The listing builds one solid part. Answer for the finished solid, in the listing's coordinates (mm). A direction names the side the tool comes from. Round coordinates to 2 decimals unless told otherwise and drop trailing zeros. Write each loop counter-clockwise with the first axis right and the second up, starting at its lowest first coordinate (ties: lowest second). Pieces come first, ordered by that corner, then holes. Notation, with made-up numbers: (63, -23) - (119, -23) arc R17 cw to (119, -1) - close; hole circle Ø2 at (-2, -23.75). An arc over 180 degrees is marked (long way). Return JSON: item names as keys, results as strings. Group by question number.
(1) Section C-C, the plane y = -91 is taken. Write down the section's boundary in (x, z), then the cut area to 3 significant figures.
(2) Each of these flat-tipped pins is pushed along its axis until it touches: pin 1 (3 mm diameter, centred on y = -12.5, z = 4.5, fed in from -X); pin 2 (3 mm diameter, centred on y = 19.5, z = 2, fed in from +X); pin 3 (6 mm diameter, centred on x = -26.5, y = -35, fed in from -Z); pin 4 (1.9 mm diameter, centred on x = -18, z = 4.5, fed in from +Y). Where does it stop, or does it pass through?
(3) Section D-D, the plane x = 32.5 is taken. Write down the section's boundary in (y, z).
(4) Section B-B, the plane x = 0 is taken. Write down the section's boundary in (y, z) (3 decimals).
(5) Find the intervals of material crossed by line 1 along X through (y, z) = (7, 3.5) (3 decimals); line 2 along X through (y, z) = (20.5, 3.25) (3 decimals); line 3 along Y through (x, z) = (110, 2), in increasing order. Write a range as [from, to].
(6) Section A-A, the plane z = 3.75 is taken. Write down the section's boundary in (x, y) (3 decimals), then the cut area to 3 significant figures.
(7) Which of the six approach directions +Z, -Z, +X, -X, +Y, -Y give full straight-line access (tool end or side, diameter ignored) to faces 1 (the flat face through (-3.175, -14, 3)), 2 (the flat face through (-2, 30, 6.35))?
(8) Determine the mould class of faces 3 (the cylindrical face through (-27.53, -123.98, 3.13)), 4 (the cylindrical face through (-28.574, -0.07, 3.131)), 5 (the flat face through (-2, 30, 0)) for opening direction Y: +Y half, -Y half, draft (parallel to the pull), parting line (faces both ways), or undercut.
```python
from build123d import *

# Parameters (mm, degrees)
F0_R     = 127
F1_DEPTH = 6.35


with BuildPart() as f1:
    # F0 (on Top) → F1 (new body)
    with BuildSketch(Plane.XY):
        Circle(F0_R)
        with BuildLine():
            Line((-3.175, -25.4), (-3.175, -3.175))
            Line((-3.175, -3.175), (-25.4, -3.175))
            ThreePointArc((-25.4, -3.175), (-28.575, 0), (-25.4, 3.175))
            Line((-25.4, 3.175), (-3.175, 3.175))
            Line((-3.175, 3.175), (-3.175, 25.4))
            ThreePointArc((-3.175, 25.4), (0, 28.575), (3.175, 25.4))
            Line((3.175, 25.4), (3.175, 3.175))
            Line((3.175, 3.175), (25.4, 3.175))
            ThreePointArc((25.4, 3.175), (28.575, 0), (25.4, -3.175))
            Line((25.4, -3.175), (3.175, -3.175))
            Line((3.175, -3.175), (3.175, -25.4))
            ThreePointArc((3.175, -25.4), (0, -28.575), (-3.175, -25.4))
        make_face(mode=Mode.SUBTRACT)
    extrude(amount=F1_DEPTH)


solid = f1.part
```
Working result:
{
 "1": {"outline": "(-88.59, 0) - (88.59, 0) - (88.59, 6.35) - (-88.59, 6.35) - close", "area": "1,130 mm^2"},
 "2": {"pin 1": "stops at x = -126.52", "pin 2": "stops at x = 125.72", "pin 3": "stops at z = 0", "pin 4": "stops at y = 125.85"},
 "3": {"outline": "(-122.77, 0) - (122.77, 0) - (122.77, 6.35) - (-122.77, 6.35) - close"},
 "4": {"outline": "(-127, 0) - (-28.575, 0) - (-28.575, 6.35) - (-127, 6.35) - close; (28.575, 0) - (127, 0) - (127, 6.35) - (28.575, 6.35) - close"},
 "5": {"line 1": "x = [-126.807, -3.175], [3.175, 126.807]", "line 2": "x = [-125.335, -3.175], [3.175, 125.335]", "line 3": "y = [-63.47, 63.47]"},
 "6": {"outline": "circle Ø254 at (0, 0); hole (-25.4, -3.175) - (-3.175, -3.175) - (-3.175, -25.4) arc R3.175 ccw to (3.175, -25.4) - (3.175, -3.175) - (25.4, -3.175) arc R3.175 ccw to (25.4, 3.175) - (3.175, 3.175) - (3.175, 25.4) arc R3.175 ccw to (-3.175, 25.4) - (-3.175, 3.175) - (-25.4, 3.175) arc R3.175 ccw to start", "area": "50,000 mm^2"},
 "7": {"face 1": "+Z, -Z", "face 2": "+Z, +X, -X, +Y, -Y"},
 "8": {"face 3": "parting line", "face 4": "undercut", "face 5": "draft"}
}
